Part print with two shaded views. Sizes in mm from the minimum x, y, z corner. A direction names the side the tool comes from. Coordinates: 2 decimals unless noted, no trailing zeros. Order: outer loops, then holes, each group sorted by start corner. A loop starts at its lowest first (then second) coordinate and runs counter-clockwise, first axis right, second up. Notation, with made-up numbers: (5.5, 34) - (43.5, 34) arc R22 cw to (43.5, 52) - close; hole circle Ø1 at (-12.75, 62.25). An arc over 180 degrees is marked (long way). Return JSON: item names as keys, results as strings.
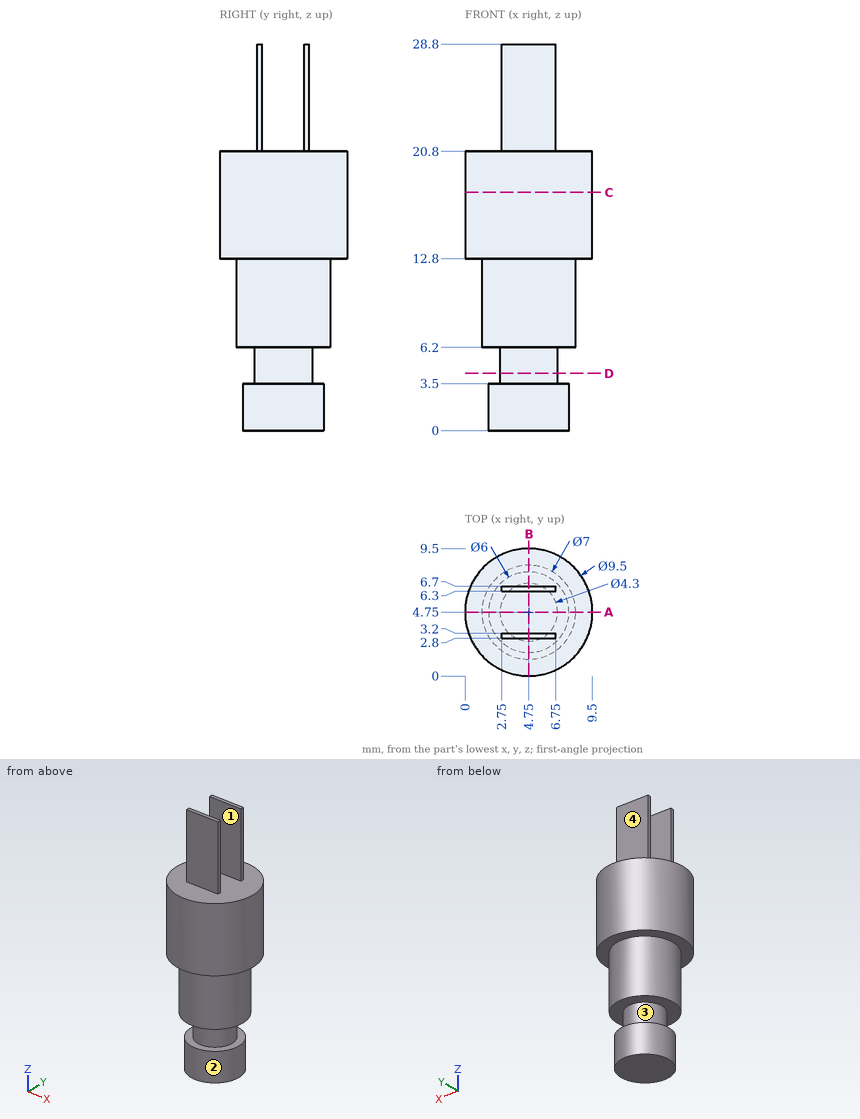
Item 1: Band-saw the part on B-B, the plane x = 4.75. List the corners of the cut face in (y, z).
Findings below:
{"outline": "(0, 12.8) - (1.25, 12.8) - (1.25, 6.2) - (2.6, 6.2) - (2.6, 3.5) - (1.75, 3.5) - (1.75, 0) - (7.75, 0) - (7.75, 3.5) - (6.9, 3.5) - (6.9, 6.2) - (8.25, 6.2) - (8.25, 12.8) - (9.5, 12.8) - (9.5, 20.8) - (6.7, 20.8) - (6.7, 28.8) - (6.3, 28.8) - (6.3, 20.8) - (3.2, 20.8) - (3.2, 28.8) - (2.8, 28.8) - (2.8, 20.8) - (0, 20.8) - close"}
Item 2: Wall check: L1, parallel to Y at x = 5.75, z = 23.5; L2, parallel to Z at x = 2, y = 5; L3, parallel to Z at x = 2.5, y = 1.25. Give the ranges that are in metal, low to high. Write a range as [from, to].
Findings below:
{"L1": "y = [2.8, 3.2], [6.3, 6.7]", "L2": "z = [0, 3.5], [6.2, 20.8]", "L3": "z = [12.8, 20.8]"}
Item 3: Band-saw the part on D-D, the plane z = 4.25. List the corners of the cut face in (x, y), then the cut area to 3 significant figures.
Findings below:
{"outline": "circle Ø4.3 at (4.75, 4.75)", "area": "14.5 mm²"}
Item 4: Band-saw the part on C-C, the plane z = 17.75. List the corners of the cut face in (x, y), then the cut area to 3 significant figures.
Findings below:
{"outline": "circle Ø9.5 at (4.75, 4.75)", "area": "70.9 mm²"}
Item 5: Band-saw the part on A-A, the plane y = 4.75. List the corners of the cut face in (x, z), then the cut area to 3 significant figures.
Findings below:
{"outline": "(0, 12.8) - (1.25, 12.8) - (1.25, 6.2) - (2.6, 6.2) - (2.6, 3.5) - (1.75, 3.5) - (1.75, 0) - (7.75, 0) - (7.75, 3.5) - (6.9, 3.5) - (6.9, 6.2) - (8.25, 6.2) - (8.25, 12.8) - (9.5, 12.8) - (9.5, 20.8) - (0, 20.8) - close", "area": "155 mm²"}
Item 6: Which spindle directions (+Z, -Z, +X, -X, +Y, -Y) get a long thin tool onto all of the face, cutting with end or side? Do the marked faces 1, 2, 3 and 4. Say none if no direction does.
Findings below:
{"face 1": "+Z, +X, -X", "face 2": "-Z", "face 3": "none", "face 4": "+Z, +X, -X, +Y"}
Item 7: Drop flat-ended pins along their axis: P1, Ø2, axis at x = 4.5, z = 25, coming from the +Y side; P2, Ø1.2, axis at x = 5, z = 26, coming from the -Y side; P3, Ø4, axis at y = 5.5, z = 23, coming from the -X side; P4, Ø3.5, axis at x = 3.5, y = 6, coming from the -Z side. Give the stop position or say it passes through.
Findings below:
{"P1": "stops at y = 6.7", "P2": "stops at y = 2.8", "P3": "stops at x = 2.75", "P4": "stops at z = 0"}
